Input: part model. Units: mm. Frame: model coordinates. Face numbers are marked on the shaded views. A direction names the side the tool comes from. Coordinates: 2 decimals unless noted, no trailing zeros. Loops run counter-clockwise (first coordinate to the right, second up) from the corner with the lowest first, then second, coordinate; pieces in that order, holes last. Notation, with made-up numbers: M -37,-38 L 15,-38 A19 ccw 15,-28 Z; hole C 19,-10.5 d5. An arc over 180 degrees is marked long. Use a Markdown table: item, result. Add a question column.
1. Section D-D on y = -53. Output: boundary loops of the cut face in (x, z).
2. Section B-B on x = 73. Output: boundary loops of the cut face in (y, z), then the cut area to 3 significant figures.
3. Line query: L1, parallel to Z at x = 64.5, y = -23.5; L2, parallel to Z at x = 67, y = -17; L3, parallel to Z at x = 76, y = -9. Output: solid intervals per line, ascending. Write a range as [from, to].
4. Draft query along Z for the marked faces 1, 2 and 3. Return one class per face: +Z half, -Z half, draft (parallel to the pull), parting line (faces both ways), or undercut.
5. Section A-A on y = -40. Output: boundary loops of the cut face in (x, z).
6. Section C-C on z = 81.5. Output: boundary loops of the cut face in (x, y).
7. Pin query (flat end, axial travel): pin 1 (6 mm diameter, centred on y = -64, z = 76, fed in from -X); pin 2 (12 mm diameter, centred on y = -9, z = 49.5, fed in from -X); pin 3 (2 mm diameter, centred on x = 32.5, z = 58.5, fed in from +Y); pin 4 (12 mm diameter, centred on y = -28.5, z = 59.5, fed in from +X). Return the tip coordinate at first contact, or that it passes through.
8. Set-up query: the marked faces 4 and 5. Return all of +Z, -Z, +X, -X, +Y, -Y with unobstructed straight access to the full face (end or side cutting, diameter ignored); none if empty.
```python
from build123d import *

# Parameters (mm, degrees)
SKETCH_1_W      = 80
SKETCH_1_H      = 80
EXTRUDE_1_DEPTH = 60
FILLET_1_R      = 10
SKETCH_2_R      = 25
EXTRUDE_2_DEPTH = 10
SKETCH_3_R      = 30
EXTRUDE_3_DEPTH = 17


with BuildPart() as part:
    # 스케치1 → 보스-돌출1 (new body)
    with BuildSketch(Plane.XY):
        with Locations((40, -40)):
            Rectangle(SKETCH_1_W, SKETCH_1_H)
    extrude(amount=EXTRUDE_1_DEPTH)

    # 필렛1
    fillet_1_edges = [part.edges().sort_by_distance(p)[0] for p in [
        (80, -40, 60),
        (40, 0, 60),
        (0, -40, 60),
        (40, 0, 0),
        (80, -40, 0),
        (40, -80, 0),
        (0, -40, 0),
        (40, -80, 60),
        (0, 0, 30),
        (80, 0, 30),
        (80, -80, 30),
        (0, -80, 30),
    ]]
    fillet(fillet_1_edges, radius=FILLET_1_R)

    # 스케치2 → 보스-돌출2 (add)
    with BuildSketch(Plane.XY.offset(60)):
        with Locations((41.207439788, -40)):
            Circle(SKETCH_2_R)
    extrude(amount=EXTRUDE_2_DEPTH)

    # 스케치3 → 보스-돌출3 (add)
    with BuildSketch(Plane.XY.offset(70)):
        with Locations((41.207439788, -40)):
            Circle(SKETCH_3_R)
    extrude(amount=EXTRUDE_3_DEPTH)


solid = part.part
```
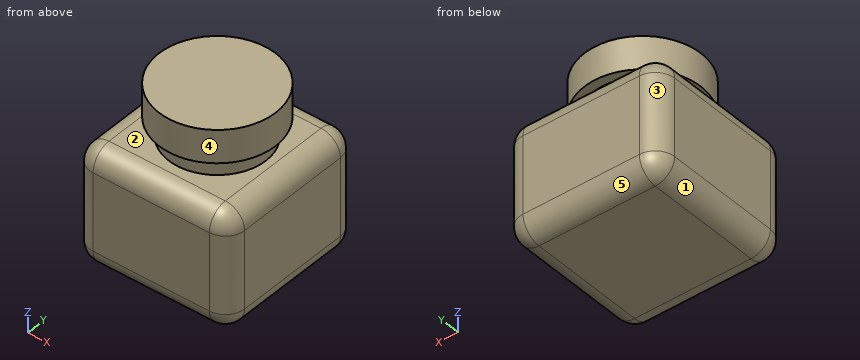
Answers below:
| question | item | result |
|---|---|---|
| 1 | outline | M 0,10 A10 ccw 10,0 L 70,0 A10 ccw 80,10 L 80,50 A10 ccw 70,60 L 62.56,60 L 62.56,70 L 68.24,70 L 68.24,87 L 14.17,87 L 14.17,70 L 19.85,70 L 19.85,60 L 10,60 A10 ccw 0,50 Z |
| 2 | outline | M -79.54,10 A9.54 ccw -70,0.46 L -10,0.46 A9.54 ccw -0.46,10 L -0.46,50 A9.54 ccw -10,59.54 L -70,59.54 A9.54 ccw -79.54,50 Z |
| 2 | area | 4,590 mm² |
| 3 | L1 | z = [0, 60], [70, 87] |
| 3 | L2 | z = [0, 60] |
| 3 | L3 | z = [2.06, 57.94] |
| 4 | face 1 | -Z half |
| 4 | face 2 | undercut |
| 4 | face 3 | draft |
| 5 | outline | M 0,10 A10 ccw 10,0 L 70,0 A10 ccw 80,10 L 80,50 A10 ccw 70,60 L 66.21,60 L 66.21,70 L 71.21,70 L 71.21,87 L 11.21,87 L 11.21,70 L 16.21,70 L 16.21,60 L 10,60 A10 ccw 0,50 Z |
| 6 | outline | C 41.21,-40 d60 |
| 7 | pin 1 | stops at x = 19.78 |
| 7 | pin 2 | stops at x = 0 |
| 7 | pin 3 | stops at y = -3.39 |
| 7 | pin 4 | stops at x = 79.37 |
| 8 | face 4 | +Z |
| 8 | face 5 | -Z, +X, -X, +Y |
